The model under review builds one solid part; all positions refer to its coordinate system, in mm. Face numbers are marked on the shaded views. Give positions to 0.01 mm unless a question says otherwise; leave off trailing zeros. Order: outer loops, then holes, each group sorted by start corner. A loop starts at its lowest first (then second) coordinate and runs counter-clockwise, first axis right, second up.
```python
from build123d import *

# Parameters (mm, degrees)
F0_R     = 9.525
F1_DEPTH = 25.4
F3_DEPTH = 25.401
F4_DEPTH = 11.0998


with BuildPart() as f1:
    # F0 (on Front) → F1 (new body)
    with BuildSketch(Plane.XZ):
        Circle(F0_R)
    extrude(amount=F1_DEPTH)

    # F2 (on face) → F3 (cut, through all)
    with BuildSketch(Plane.XZ.offset(25.4)):
        with BuildLine():
            ThreePointArc((-4.7625, 0), (-3.367596, -3.367596), (0, -4.7625))
            ThreePointArc((0, -4.7625), (3.367596, -3.367596), (4.7625, 0))
            ThreePointArc((4.7625, 0), (3.367596, 3.367596), (0, 4.7625))
            ThreePointArc((0, 4.7625), (-3.367596, 3.367596), (-4.7625, 0))
        make_face()
    extrude(amount=-F3_DEPTH, mode=Mode.SUBTRACT)

    # F2 (on face) → F4 (cut)
    with BuildSketch(Plane.XZ.offset(25.4)):
        with BuildLine():
            Line((0, -4.7625), (4.7625, -4.7625))
            Line((4.7625, -4.7625), (4.7625, 0))
            ThreePointArc((4.7625, 0), (3.367596, -3.367596), (0, -4.7625))
        make_face()
        with BuildLine():
            Line((-4.7625, -4.7625), (0, -4.7625))
            ThreePointArc((0, -4.7625), (-3.367596, -3.367596), (-4.7625, 0))
            Line((-4.7625, 0), (-4.7625, -4.7625))
        make_face()
        with BuildLine():
            ThreePointArc((0, 4.7625), (3.367596, 3.367596), (4.7625, 0))
            Line((4.7625, 0), (4.7625, 4.7625))
            Line((4.7625, 4.7625), (0, 4.7625))
        make_face()
        with BuildLine():
            Line((-4.7625, 4.7625), (-4.7625, 0))
            ThreePointArc((-4.7625, 0), (-3.367596, 3.367596), (0, 4.7625))
            Line((0, 4.7625), (-4.7625, 4.7625))
        make_face()
    extrude(amount=-F4_DEPTH, mode=Mode.SUBTRACT)


solid = f1.part
```
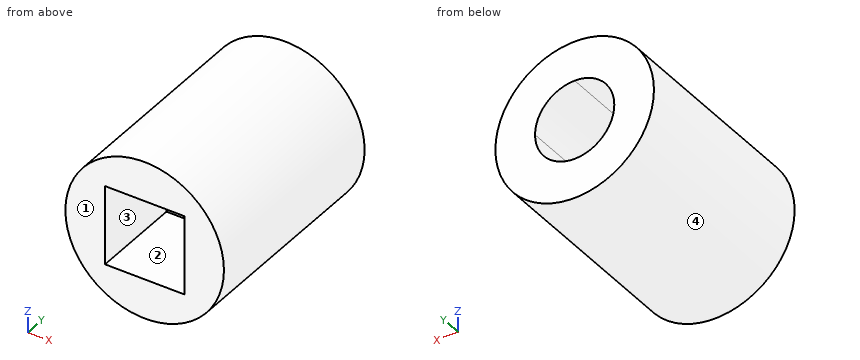
Item 1: Take a section at C-C (z = -3.75). Give the boundary of the cut face in (x, y).
Values found:
outline: (-8.76, -25.4) - (-4.76, -25.4) - (-4.76, -14.3) - (-2.94, -14.3) - (-2.94, 0) - (-8.76, 0) - close; (2.94, -14.3) - (4.76, -14.3) - (4.76, -25.4) - (8.76, -25.4) - (8.76, 0) - (2.94, 0) - close
Item 2: Clearance check with flat-ended pins moving along their axes: pin 1 Ø1.5 at (x, y) = (3.5, -18.5) entering from +Z; pin 2 Ø1 at (x, y) = (6, -21.5) entering from -Z; pin 3 Ø6 at (y, z) = (-17, 6) entering from -X; pin 4 Ø2.5 at (x, z) = (1.5, -1.5) entering from -Y. State where each tip first meets the part, or that it passes through.
Values found:
pin 1: stops at z = 9.12
pin 2: stops at z = -7.78
pin 3: stops at x = -9.04
pin 4: passes through
Item 3: For line 1 (X direction, y = -22.25, z = -8.25); line 2 (X direction, y = -9.75, z = 3.75); line 3 (Z direction, x = 1, y = -9.5), list the stretches that pass through material, from the lowest coordinate up.
Values found:
line 1: x = -4.76 to 4.76
line 2: x = -8.76 to -2.94, 2.94 to 8.76
line 3: z = -9.47 to -4.66, 4.66 to 9.47
Item 4: Draft analysis for pull direction X (two halves, no side actions). For the marked faces 1, 2, 3 and 4, state which applies: released by +X, released by -X, zero draft, split by the parting line, or undercut.
Values found:
face 1: zero draft
face 2: undercut
face 3: undercut
face 4: split by the parting line
